from build123d import *

# Parameters (mm, degrees)
BOSS_EXTRUDE4_DEPTH = 3
SKETCH4_R           = 4
CUT_EXTRUDE1_DEPTH  = 80.909323611
SKETCH5_R           = 4
BOSS_EXTRUDE5_DEPTH = 8


with BuildPart() as part:
    # Sketch1 → Boss-Extrude4 (new body)
    with BuildSketch(Plane.XY):
        with BuildLine():
            Line((0, 7.5), (72, 7.5))
            ThreePointArc((72, 7.5), (79.5, 0), (72, -7.5))
            Line((72, -7.5), (0, -7.5))
            ThreePointArc((0, -7.5), (-7.5, 0), (0, 7.5))
        make_face()
    extrude(amount=BOSS_EXTRUDE4_DEPTH)

    # Sketch4 → Cut-Extrude1 (cut, through all)
    with BuildSketch(Plane.XY.offset(3)):
        Circle(SKETCH4_R)
    extrude(amount=-CUT_EXTRUDE1_DEPTH, mode=Mode.SUBTRACT)

    # Sketch5 → Boss-Extrude5 (add)
    with BuildSketch(Plane.XY.offset(3)):
        with Locations((72, 0)):
            Circle(SKETCH5_R)
    extrude(amount=BOSS_EXTRUDE5_DEPTH)


solid = part.part
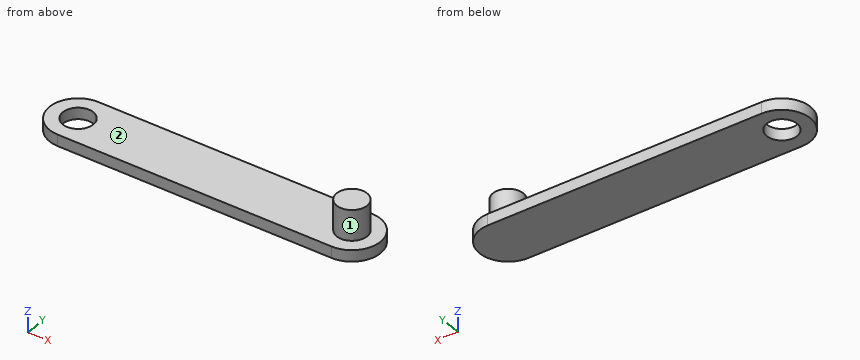
The listing builds one solid part. Answer for the finished solid, in the listing's coordinates (mm). Face numbers are marked on the shaded views. Give positions to 0.01 mm unless a question says otherwise; leave off trailing zeros. Write each loop counter-clockwise with the first axis right and the second up, starting at its lowest first coordinate (ties: lowest second). Pieces come first, ordered by that corner, then holes. Notation, with made-up numbers: (74, -9.75) -> (102, -9.75) arc R19 cw to (102, 8.25) -> close; hole circle Ø6 at (0.25, 24.5). An arc over 180 degrees is marked (long way). Use a Markdown table: item, result.
(1) Find the intervals of material crossed by probe 1 along Y at (x, z) = (0, 0.85); probe 2 along Z at (x, y) = (52.5, -2.75); probe 3 along X at (y, z) = (-1.75, 1.75), in increasing order. Write a range as from..to.
Return value:
| item | result |
|---|---|
| probe 1 | -7.5..-4, 4..7.5 |
| probe 2 | 0..3 |
| probe 3 | -7.29..-3.6, 3.6..79.29 |
(2) Section A-A, the plane y = 0 is taken. Determine the outline of the cut face in (x, z).
Return value:
| item | result |
|---|---|
| outline | (-7.5, 0) -> (-4, 0) -> (-4, 3) -> (-7.5, 3) -> close; (4, 0) -> (79.5, 0) -> (79.5, 3) -> (76, 3) -> (76, 11) -> (68, 11) -> (68, 3) -> (4, 3) -> close |
(3) Determine the mould class of the marked faces 1 and 2 for opening direction Y: released by +Y, released by -Y, zero draft, split by the parting line, or undercut.
Return value:
| item | result |
|---|---|
| face 1 | split by the parting line |
| face 2 | zero draft |
(4) Section D-D, the plane z = 6.75 is taken. Determine the outline of the cut face in (x, y), then the cut area to 3 significant figures.
Return value:
| item | result |
|---|---|
| outline | circle Ø8 at (72, 0) |
| area | 50.3 mm2 |
(5) Flat-ended cylindrical pins translate along their axes: P1, Ø1.5, axis at y = 3.5, z = 8.5, coming from the +X side; P2, Ø1, axis at y = -5, z = 1, coming from the -X side; P3, Ø1, axis at y = -2.5, z = 4, coming from the +X side. Find the tip coordinate at first contact, or state that the pin passes through.
Return value:
| item | result |
|---|---|
| P1 | x = 74.9 |
| P2 | x = -6 |
| P3 | x = 75.46 |
(6) Section B-B, the plane z = 1.5 is taken. Determine the outline of the cut face in (x, y), then the cut area to 3 significant figures.
Return value:
| item | result |
|---|---|
| outline | (0, -7.5) -> (72, -7.5) arc R7.5 ccw to (72, 7.5) -> (0, 7.5) arc R7.5 ccw to start; hole circle Ø8 at (0, 0) |
| area | 1,210 mm2 |
(7) Section C-C, the plane x = 60 is taken. Determine the outline of the cut face in (y, z), then the cut area to 3 significant figures.
Return value:
| item | result |
|---|---|
| outline | (-7.5, 0) -> (7.5, 0) -> (7.5, 3) -> (-7.5, 3) -> close |
| area | 45.0 mm2 |
